```python
from build123d import *

# Parameters (mm, degrees)
SKETCH3_W                                = 71
SKETCH3_H                                = 60
BOSS_EXTRUDE2_DEPTH                      = 57
SKETCH4_W                                = 5
SKETCH4_H                                = 15.5
BOSS_EXTRUDE4_DEPTH                      = 52
SKETCH8_W                                = 5
SKETCH8_H                                = 15.5
BOSS_EXTRUDE5_DEPTH                      = 4
M3_CLEARANCE_HOLE1_D                     = 3.4
M3_CLEARANCE_HOLE1_DEPTH                 = 60
CHAMFER1_SIZE                            = 3
CHAMFER1_OF_MIRROR1_SIZE                 = 3
SKETCH12_W                               = 7
SKETCH12_H                               = 23.5
BOSS_EXTRUDE6_DEPTH                      = 62
CUT_EXTRUDE1_REACH                       = 89.267
SKETCH13_W                               = 20
SKETCH13_H                               = 41
M4_CLEARANCE_HOLE3_D                     = 4.5
M4_CLEARANCE_HOLE3_DEPTH                 = 7
SKETCH17_W                               = 21
SKETCH17_H                               = 41
CUT_EXTRUDE2_DEPTH                       = 30
CUT_EXTRUDE4_DEPTH                       = 21
M4_CLEARANCE_HOLE4_AT_2_COUNT            = 2
M4_CLEARANCE_HOLE4_AT_2_PITCH            = 10
M4_CLEARANCE_HOLE4_AT_3_COUNT            = 2
M4_CLEARANCE_HOLE4_AT_3_PITCH            = 50.009999
M4_CLEARANCE_HOLE4_AT_4_COUNT            = 2
M4_CLEARANCE_HOLE4_AT_4_PITCH            = 49
CUT_EXTRUDE3_DEPTH                       = 4
SHELL1_START                             = -11
SHELL1_DEPTH                             = 42
SKETCH22_W                               = 15
SKETCH22_H                               = 15
BOSS_EXTRUDE7_DEPTH                      = 10
CBORE_FOR_M4_PAN_HEAD_SCREW1_D           = 4.5
CBORE_FOR_M4_PAN_HEAD_SCREW1_CBORE_D     = 9
CBORE_FOR_M4_PAN_HEAD_SCREW1_CBORE_DEPTH = 3.1
CHAMFER2_SIZE                            = 4
CHAMFER2_OF_MIRROR3_SIZE                 = 4
CHAMFER3_SIZE                            = 5
CHAMFER4_SIZE                            = 5


# Read off the part's stored shape, not the designer's step: Shell1
with BuildPart() as part:
    # Sketch3 → Boss-Extrude2 (new body)
    with BuildSketch(Plane(origin=(0, 0, 0), x_dir=(1, 0, 0), z_dir=(0, 1, 0))):
        with Locations((0, -10)):
            Rectangle(SKETCH3_W, SKETCH3_H)
    extrude(amount=BOSS_EXTRUDE2_DEPTH)

    # Sketch4 → Boss-Extrude4 (add)
    with BuildSketch(Plane(origin=(0, 0, 0), x_dir=(1, 0, 0), z_dir=(0, 1, 0))):
        with Locations((-27.5, 27.75)):
            Rectangle(SKETCH4_W, SKETCH4_H)
    boss_extrude4 = extrude(amount=BOSS_EXTRUDE4_DEPTH)

    # Sketch8 → Boss-Extrude5 (add)
    with BuildSketch(Plane(origin=(0, 52, 0), x_dir=(1, 0, 0), z_dir=(0, 1, 0))):
        with Locations((-27.5, 27.75)):
            Rectangle(SKETCH8_W, SKETCH8_H)
    boss_extrude5 = extrude(amount=BOSS_EXTRUDE5_DEPTH)

    # M3 Clearance Hole1
    with Locations(Plane.ZY.offset(30)):
        with Locations((-31.5, 22), (-31.5, 52)):
            m3_clearance_hole1 = Hole(M3_CLEARANCE_HOLE1_D / 2, depth=M3_CLEARANCE_HOLE1_DEPTH)

    # Chamfer1
    chamfer1_edges = [part.edges().sort_by_distance(p)[0] for p in [
        (-27.5, 0, -35.5),
        (-27.5, 56, -35.5),
    ]]
    chamfer(chamfer1_edges, length=CHAMFER1_SIZE)

    # Mirror1: Boss-Extrude4, Boss-Extrude5, M3 Clearance Hole1 across plane
    add(boss_extrude4.mirror(Plane(origin=(0, 0, 0), x_dir=(0, 0, 1), z_dir=(1, 0, 0))))
    add(boss_extrude5.mirror(Plane(origin=(0, 0, 0), x_dir=(0, 0, 1), z_dir=(1, 0, 0))))
    add(m3_clearance_hole1.mirror(Plane(origin=(0, 0, 0), x_dir=(0, 0, 1), z_dir=(1, 0, 0))), mode=Mode.SUBTRACT)

    # Chamfer1 of Mirror1
    chamfer1_of_mirror1_edges = [part.edges().sort_by_distance(p)[0] for p in [
        (27.5, 0, -35.5),
        (27.5, 56, -35.5),
    ]]
    chamfer(chamfer1_of_mirror1_edges, length=CHAMFER1_OF_MIRROR1_SIZE)

    # Sketch12 → Boss-Extrude6 (add)
    with BuildSketch(Plane(origin=(0, 0, 0), x_dir=(1, 0, 0), z_dir=(0, 1, 0))):
        with Locations((-4.35, 31.75)):
            Rectangle(SKETCH12_W, SKETCH12_H)
    extrude(amount=BOSS_EXTRUDE6_DEPTH)

    # Sketch13 → Cut-Extrude1 (cut, up to next)
    with BuildSketch(Plane.ZY.offset(7.85), mode=Mode.PRIVATE) as cut_extrude1_sk1:
        with Locations((-31.5, 32)):
            Rectangle(SKETCH13_W, SKETCH13_H)
    cut_extrude1_tool1 = extrude(cut_extrude1_sk1.sketch, amount=-CUT_EXTRUDE1_REACH, mode=Mode.PRIVATE) & part.part
    add(cut_extrude1_tool1.solids().sort_by_distance((-7.85, 32, -31.5))[0], mode=Mode.SUBTRACT)

    # M4 Clearance Hole3
    with Locations(Plane.ZY.offset(7.85)):
        with Locations((-36.5, 8), (-26.5, 8), (-36.5, 56), (-26.5, 56)):
            Hole(M4_CLEARANCE_HOLE3_D / 2, depth=M4_CLEARANCE_HOLE3_DEPTH)

    # Sketch17 → Cut-Extrude2 (cut)
    with BuildSketch(Plane(origin=(0, 57, 0), x_dir=(1, 0, 0), z_dir=(0, 1, 0))):
        with Locations((-25, -10.5)):
            Rectangle(SKETCH17_W, SKETCH17_H)
        with Locations((25, -10.5)):
            Rectangle(SKETCH17_W, SKETCH17_H)
    extrude(amount=-CUT_EXTRUDE2_DEPTH, mode=Mode.SUBTRACT)

    # Sketch21 → Cut-Extrude4 (cut)
    with BuildSketch(Plane.ZY.offset(35.5)):
        Polygon((-10, 27), (-15, 27), (-15, 37), (-10, 42), align=None)
    cut_extrude4 = extrude(amount=-CUT_EXTRUDE4_DEPTH, mode=Mode.SUBTRACT)

    # Sketch18 → M4 Clearance Hole4 (revolve, cut)
    with BuildSketch(Plane(origin=(-30, 57, -14), x_dir=(0, 0, 1), z_dir=(1, 0, 0))):
        Polygon((0, 0), (0, 16.351936393), (2.25, 15), (2.25, 0), align=None)
    m4_clearance_hole4 = revolve(axis=Axis((-30, 63.35, -14), (0, -1, 0)), mode=Mode.SUBTRACT)

    # M4 Clearance Hole4 at 2: M4 Clearance Hole4 ×2
    with Locations(*[(i * M4_CLEARANCE_HOLE4_AT_2_PITCH, 0, 0) for i in range(1, M4_CLEARANCE_HOLE4_AT_2_COUNT)]):
        add(m4_clearance_hole4, mode=Mode.SUBTRACT)

    # M4 Clearance Hole4 at 3: M4 Clearance Hole4 ×2
    with Locations(*[Vector(0.19996001199600155, 0, 0.9798040587804069) * (i * M4_CLEARANCE_HOLE4_AT_3_PITCH) for i in range(1, M4_CLEARANCE_HOLE4_AT_3_COUNT)]):
        add(m4_clearance_hole4, mode=Mode.SUBTRACT)

    # M4 Clearance Hole4 at 4: M4 Clearance Hole4 ×2
    with Locations(*[(0, 0, i * M4_CLEARANCE_HOLE4_AT_4_PITCH) for i in range(1, M4_CLEARANCE_HOLE4_AT_4_COUNT)]):
        add(m4_clearance_hole4, mode=Mode.SUBTRACT)

    # Sketch20 → Cut-Extrude3 (cut)
    with BuildSketch(Plane(origin=(0, 52, 0), x_dir=(1, 0, 0), z_dir=(0, 1, 0))):
        Polygon((-34.272391992, 14), (-34.272391992, 10), (-25.727608008, 10), (-25.727608008, 14), (-27.863804004, 17.7), (-32.136195996, 17.7), align=None)
        Polygon((-24.272391992, 10), (-24.272391992, 14), (-22.136195996, 17.7), (-17.863804004, 17.7), (-15.727608008, 14), (-15.727608008, 10), align=None)
        Polygon((-15.727608008, -35), (-15.727608008, -31), (-24.272391992, -31), (-24.272391992, -35), (-22.136195996, -38.7), (-17.863804004, -38.7), align=None)
        Polygon((-25.727608008, -31), (-25.727608008, -35), (-27.863804004, -38.7), (-32.136195996, -38.7), (-34.272391992, -35), (-34.272391992, -31), align=None)
    cut_extrude3 = extrude(amount=-CUT_EXTRUDE3_DEPTH, mode=Mode.SUBTRACT)

    # Mirror2: Cut-Extrude4, M4 Clearance Hole4, Cut-Extrude3 across plane
    add(cut_extrude4.mirror(Plane(origin=(0, 0, 0), x_dir=(0, 0, 1), z_dir=(1, 0, 0))), mode=Mode.SUBTRACT)
    add(m4_clearance_hole4.mirror(Plane(origin=(0, 0, 0), x_dir=(0, 0, 1), z_dir=(1, 0, 0))), mode=Mode.SUBTRACT)
    add(cut_extrude3.mirror(Plane(origin=(0, 0, 0), x_dir=(0, 0, 1), z_dir=(1, 0, 0))), mode=Mode.SUBTRACT)

    # Mirror2 copy 1 sketch → Mirror2 copy 1 (revolve, cut)
    with BuildSketch(Plane(origin=(20, 57, -14), x_dir=(0, 0, 1), z_dir=(-1, 0, 0))):
        Polygon((0, 0), (0, -16.351936393), (2.25, -15), (2.25, 0), align=None)
    revolve(axis=Axis((20, 63.35, -14), (0, 1, 0)), mode=Mode.SUBTRACT)

    # Mirror2 copy 2 sketch → Mirror2 copy 2 (revolve, cut)
    with BuildSketch(Plane(origin=(20, 57, 35), x_dir=(0, 0, 1), z_dir=(-1, 0, 0))):
        Polygon((0, 0), (0, -16.351936393), (2.25, -15), (2.25, 0), align=None)
    revolve(axis=Axis((20, 63.35, 35), (0, 1, 0)), mode=Mode.SUBTRACT)

    # Mirror2 copy 3 sketch → Mirror2 copy 3 (revolve, cut)
    with BuildSketch(Plane(origin=(30, 57, 35), x_dir=(0, 0, 1), z_dir=(-1, 0, 0))):
        Polygon((0, 0), (0, -16.351936393), (2.25, -15), (2.25, 0), align=None)
    revolve(axis=Axis((30, 63.35, 35), (0, 1, 0)), mode=Mode.SUBTRACT)

    # Shell1 outline → Shell1 (cut)
    with BuildSketch(Plane.XY.offset(SHELL1_START)):
        Polygon((-5.5, 18), (-26.5, 18), (-26.5, 0), (26.5, 0), (26.5, 18), (5.5, 18), (5.5, 48), (-5.5, 48), align=None)
    extrude(amount=SHELL1_DEPTH, mode=Mode.SUBTRACT)

    # Sketch22 → Boss-Extrude7 (add)
    with BuildSketch(Plane(origin=(0, 0, 0), x_dir=(1, 0, 0), z_dir=(0, 1, 0))):
        with Locations((43, 12.5)):
            Rectangle(SKETCH22_W, SKETCH22_H)
        with Locations((43, -32.5)):
            Rectangle(SKETCH22_W, SKETCH22_H)
    boss_extrude7 = extrude(amount=BOSS_EXTRUDE7_DEPTH)

    # CBORE for M4 Pan Head Screw1 (through all)
    with Locations(Plane(origin=(0, 10, 0), x_dir=(1, 0, 0), z_dir=(0, 1, 0))):
        with Locations((43, 12.5), (43, -32.5)):
            cbore_for_m4_pan_head_screw1 = CounterBoreHole(CBORE_FOR_M4_PAN_HEAD_SCREW1_D / 2, CBORE_FOR_M4_PAN_HEAD_SCREW1_CBORE_D / 2, CBORE_FOR_M4_PAN_HEAD_SCREW1_CBORE_DEPTH)

    # Chamfer2
    chamfer2_edges = [part.edges().sort_by_distance(p)[0] for p in [
        (50.5, 5, 40),
        (50.5, 5, 25),
        (50.5, 5, -5),
        (50.5, 5, -20),
    ]]
    chamfer(chamfer2_edges, length=CHAMFER2_SIZE)

    # Mirror3: Boss-Extrude7, CBORE for M4 Pan Head Screw1 across plane
    add(boss_extrude7.mirror(Plane(origin=(0, 0, 0), x_dir=(0, 0, 1), z_dir=(1, 0, 0))))
    add(cbore_for_m4_pan_head_screw1.mirror(Plane(origin=(0, 0, 0), x_dir=(0, 0, 1), z_dir=(1, 0, 0))), mode=Mode.SUBTRACT)

    # Chamfer2 of Mirror3
    chamfer2_of_mirror3_edges = [part.edges().sort_by_distance(p)[0] for p in [
        (-50.5, 5, 40),
        (-50.5, 5, 25),
        (-50.5, 5, -5),
        (-50.5, 5, -20),
    ]]
    chamfer(chamfer2_of_mirror3_edges, length=CHAMFER2_OF_MIRROR3_SIZE)

    # Chamfer3
    chamfer3_edges = [part.edges().sort_by_distance(p)[0] for p in [
        (-4.35, 57, -20),
    ]]
    chamfer(chamfer3_edges, length=CHAMFER3_SIZE - 0.0001)  # a hair under: the kernel refuses the full size

    # Chamfer4
    chamfer4_edges = [part.edges().sort_by_distance(p)[0] for p in [
        (-4.35, 0, -43.5),
        (-4.35, 62, -43.5),
    ]]
    chamfer(chamfer4_edges, length=CHAMFER4_SIZE)


solid = part.part
```
Read the model definition and answer for the solid it produces. Units are mm, in the model's axes. A direction names the side the tool comes from. Give positions to 0.01 mm unless a question says otherwise; leave off trailing zeros. Write each loop counter-clockwise with the first axis right and the second up, starting at its lowest first coordinate (ties: lowest second). Pieces come first, ordered by that corner, then holes. Notation, with made-up numbers: (61, 42) - (106, 42) arc R7 cw to (106, 47) - close; hole circle Ø2 at (-7, 69). An arc over 180 degrees is marked (long way). Write item = value, one per line. Start each with the question number.
Item 1: Find section C-C (x = 11.5). Give the vertices of the cut face in (y, z), then the cut area to 3 significant figures.
Item 2: Find the intervals of material crossed by probe 1 along Z at (x, y) = (43, 2.75); probe 2 along X at (y, z) = (45.9, -14); probe 3 along Z at (x, y) = (-43, 7.65), in increasing order. Write a range as [from, to].
Item 3: Each of these flat-tipped pins is pushed along its axis until it touches: P1, Ø23, axis at y = 33.5, z = -28, coming from the -X side; P2, Ø1.5, axis at y = 51, z = -21.5, coming from the -X side; P3, Ø1.5, axis at x = 7.5, y = 16, coming from the -Z side; P4, Ø8.5, axis at x = 29.5, z = 34, coming from the -Y side. Where does it stop, or does it pass through?
Item 4: The mould has two halves that part along X. Classify faces 4 (the cylindrical face through (27.47, 52.51, -33.12)), 5 (the flat face through (-4, 11.5, -32)), 6 (the flat face through (48.5, 4.9, 27)): +X half, -X half, draft (parallel to the pull), parting line (faces both ways), or undercut.
Item 5: A tool of negligible diameter and unlimited length cuts with its end or side. For faces 1 (the flat face through (39.6, 10, -15.9)), 2 (the flat face through (-30, 52, -11)), 3 (the cylindrical face through (-29.14, 54.54, -11.92)), from which of +Z, -Z, +X, -X, +Y, -Y can it reach the whole face along a straight path? Write none if from no direction.
Item 6: Find section A-A (y = 38.5). State how many separate pieces and enclosed holes the cut face has, then the cut area to 3 significant figures.
Response:
q1.outline = (0, -20) - (57, -20) - (57, 40) - (0, 40) - (0, 31) - (18, 31) - (18, -11) - (0, -11) - close
q1.area = 2,660 mm²
q2.probe_1 = [-20, -14.75], [-10.25, -5], [25, 30.25], [34.75, 40]
q2.probe_2 = [-35.5, -32.25], [-27.75, -22.25], [-17.75, 17.75], [22.25, 27.75], [32.25, 35.5]
q2.probe_3 = [-20, -17], [-8, -5], [25, 28], [37, 40]
q3.P1 = -35.5
q3.P2 = -30
q3.P3 = -20
q3.P4 = 0
q4.face_4 = draft
q4.face_5 = undercut
q4.face_6 = +X half
q5.face_1 = +Z, -Z, +X, +Y
q5.face_2 = none
q5.face_3 = +Y
q6.separate_pieces = 2
q6.enclosed_holes = 1
q6.area = 2,110 mm²
